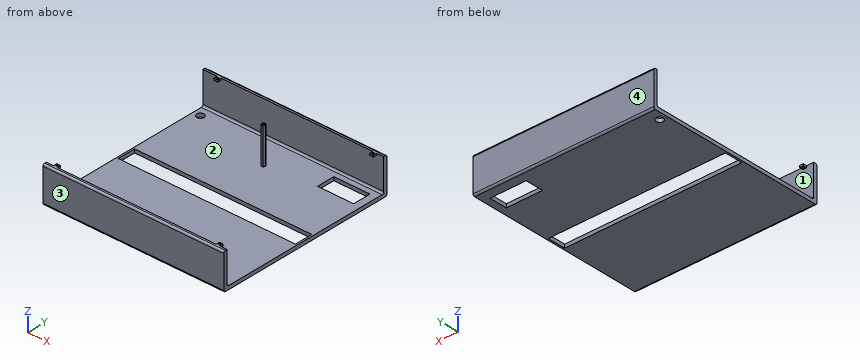
```python
from build123d import *

# Parameters (mm, degrees)
CROQUIS1_W              = 50
CROQUIS1_H              = 50
SALIENTE_EXTRUIR1_DEPTH = 10
CROQUIS2_W              = 49
CROQUIS2_H              = 5
CORTAR_EXTRUIR2_DEPTH   = 6
CROQUIS3_W              = 10
CROQUIS3_H              = 5
CORTAR_EXTRUIR3_DEPTH   = 6
CROQUIS4_R              = 1
CORTAR_EXTRUIR4_DEPTH   = 6
CROQUIS5_W              = 9
CROQUIS5_H              = 48
CORTAR_EXTRUIR5_DEPTH   = 50
CROQUIS6_W              = 1
CROQUIS6_H              = 0.5
SALIENTE_EXTRUIR2_DEPTH = 1
CROQUIS7_W              = 1
CROQUIS7_H              = 0.5
SALIENTE_EXTRUIR3_DEPTH = 1
CROQUIS9_W              = 1
CROQUIS9_H              = 0.5
SALIENTE_EXTRUIR4_DEPTH = 1
CROQUIS10_W             = 1
CROQUIS10_H             = 0.5
SALIENTE_EXTRUIR5_DEPTH = 1
SALIENTE_EXTRUIR6_DEPTH = 10
CROQUIS12_R             = 0.35
CORTAR_EXTRUIR6_DEPTH   = 9
CROQUIS13_R             = 0.25
CORTAR_EXTRUIR7_DEPTH   = 2
CROQUIS14_R             = 0.25
CORTAR_EXTRUIR8_DEPTH   = 2
CROQUIS15_R             = 0.25
CORTAR_EXTRUIR9_DEPTH   = 2
CROQUIS16_R             = 0.25
CORTAR_EXTRUIR10_DEPTH  = 2
REDONDEO5_R             = 0.5
REDONDEO6_R             = 0.5
REDONDEO7_R             = 0.5
REDONDEO8_R             = 0.5
REDONDEO9_R             = 0.5
REDONDEO10_R            = 0.5


with BuildPart() as part:
    # Croquis1 → Saliente-Extruir1 (new body)
    with BuildSketch(Plane.XY):
        Rectangle(CROQUIS1_W, CROQUIS1_H)
    extrude(amount=SALIENTE_EXTRUIR1_DEPTH)

    # Croquis2 → Cortar-Extruir2 (cut)
    with BuildSketch(Plane(origin=(0, 0, 0), x_dir=(-1, 0, 0), z_dir=(0, 0, -1))):
        Rectangle(CROQUIS2_W, CROQUIS2_H)
    extrude(amount=-CORTAR_EXTRUIR2_DEPTH, mode=Mode.SUBTRACT)

    # Croquis3 → Cortar-Extruir3 (cut)
    with BuildSketch(Plane(origin=(0, 0, 0), x_dir=(-1, 0, 0), z_dir=(0, 0, -1))):
        with Locations((-18, 19.5)):
            Rectangle(CROQUIS3_W, CROQUIS3_H)
    extrude(amount=-CORTAR_EXTRUIR3_DEPTH, mode=Mode.SUBTRACT)

    # Croquis4 → Cortar-Extruir4 (cut)
    with BuildSketch(Plane(origin=(0, 0, 0), x_dir=(-1, 0, 0), z_dir=(0, 0, -1))):
        with Locations((23, 21)):
            Circle(CROQUIS4_R)
    extrude(amount=-CORTAR_EXTRUIR4_DEPTH, mode=Mode.SUBTRACT)

    # Croquis5 → Cortar-Extruir5 (cut)
    with BuildSketch(Plane(origin=(25, 0, 0), x_dir=(0, 0, -1), z_dir=(1, 0, 0))):
        with Locations((-5.5, 0)):
            Rectangle(CROQUIS5_W, CROQUIS5_H)
    extrude(amount=-CORTAR_EXTRUIR5_DEPTH, mode=Mode.SUBTRACT)

    # Croquis6 → Saliente-Extruir2 (add)
    with BuildSketch(Plane.XZ.offset(-24)):
        with Locations((-20.5, 9.75)):
            Rectangle(CROQUIS6_W, CROQUIS6_H)
    extrude(amount=SALIENTE_EXTRUIR2_DEPTH)

    # Croquis7 → Saliente-Extruir3 (add)
    with BuildSketch(Plane.XZ.offset(-24)):
        with Locations((22.5, 9.75)):
            Rectangle(CROQUIS7_W, CROQUIS7_H)
    extrude(amount=SALIENTE_EXTRUIR3_DEPTH)

    # Croquis9 → Saliente-Extruir4 (add)
    with BuildSketch(Plane(origin=(0, -24, 0), x_dir=(1, 0, 0), z_dir=(0, 1, 0))):
        with Locations((-22.5, -9.75)):
            Rectangle(CROQUIS9_W, CROQUIS9_H)
    extrude(amount=SALIENTE_EXTRUIR4_DEPTH)

    # Croquis10 → Saliente-Extruir5 (add)
    with BuildSketch(Plane(origin=(0, -24, 0), x_dir=(1, 0, 0), z_dir=(0, 1, 0))):
        with Locations((22.5, -9.75)):
            Rectangle(CROQUIS10_W, CROQUIS10_H)
    extrude(amount=SALIENTE_EXTRUIR5_DEPTH)

    # Croquis11 → Saliente-Extruir6 (add)
    with BuildSketch(Plane.XY.offset(1)):
        Polygon((0, 15.5), (-0.288675135, 16), (-0.866025404, 16), (-1.154700538, 15.5), (-0.866025404, 15), (-0.288675135, 15), align=None)
    extrude(amount=SALIENTE_EXTRUIR6_DEPTH)

    # Croquis12 → Cortar-Extruir6 (cut)
    with BuildSketch(Plane.XY.offset(11)):
        with Locations((-0.6, 15.5)):
            Circle(CROQUIS12_R)
    extrude(amount=-CORTAR_EXTRUIR6_DEPTH, mode=Mode.SUBTRACT)

    # Croquis13 → Cortar-Extruir7 (cut)
    with BuildSketch(Plane.XY.offset(10)):
        with Locations((-20.5, 23.5)):
            Circle(CROQUIS13_R)
    extrude(amount=-CORTAR_EXTRUIR7_DEPTH, mode=Mode.SUBTRACT)

    # Croquis14 → Cortar-Extruir8 (cut)
    with BuildSketch(Plane.XY.offset(10)):
        with Locations((22.5, 23.5)):
            Circle(CROQUIS14_R)
    extrude(amount=-CORTAR_EXTRUIR8_DEPTH, mode=Mode.SUBTRACT)

    # Croquis15 → Cortar-Extruir9 (cut)
    with BuildSketch(Plane.XY.offset(10)):
        with Locations((-22.5, -23.5)):
            Circle(CROQUIS15_R)
    extrude(amount=-CORTAR_EXTRUIR9_DEPTH, mode=Mode.SUBTRACT)

    # Croquis16 → Cortar-Extruir10 (cut)
    with BuildSketch(Plane.XY.offset(10)):
        with Locations((22.5, -23.5)):
            Circle(CROQUIS16_R)
    extrude(amount=-CORTAR_EXTRUIR10_DEPTH, mode=Mode.SUBTRACT)

    # Redondeo5
    redondeo5_edges = [part.edges().sort_by_distance(p)[0] for p in [
        (0, 25, 0),
    ]]
    fillet(redondeo5_edges, radius=REDONDEO5_R)

    # Redondeo6
    redondeo6_edges = [part.edges().sort_by_distance(p)[0] for p in [
        (0, -25, 0),
    ]]
    fillet(redondeo6_edges, radius=REDONDEO6_R)

    # Redondeo7
    redondeo7_edges = [part.edges().sort_by_distance(p)[0] for p in [
        (0, 24, 1),
    ]]
    fillet(redondeo7_edges, radius=REDONDEO7_R)

    # Redondeo8
    redondeo8_edges = [part.edges().sort_by_distance(p)[0] for p in [
        (0, -24, 1),
    ]]
    fillet(redondeo8_edges, radius=REDONDEO8_R)

    # Redondeo9
    redondeo9_edges = [part.edges().sort_by_distance(p)[0] for p in [
        (0, 25, 10),
    ]]
    fillet(redondeo9_edges, radius=REDONDEO9_R)

    # Redondeo10
    redondeo10_edges = [part.edges().sort_by_distance(p)[0] for p in [
        (0, -25, 10),
    ]]
    fillet(redondeo10_edges, radius=REDONDEO10_R)


solid = part.part
```
The listing builds one solid part. Answer for the finished solid, in the listing's coordinates (mm). Face numbers are marked on the shaded views. Give positions to 0.01 mm unless a question says otherwise; leave off trailing zeros. Order: outer loops, then holes, each group sorted by start corner. A loop starts at its lowest first (then second) coordinate and runs counter-clockwise, first axis right, second up.
Item 1: The part is cut by section B-B, the plane z = 4.75. Give the vertices of the cut face in (x, y).
From the geometry:
outline: (-25, -25) - (25, -25) - (25, -24) - (-25, -24) - close; (-25, 24) - (25, 24) - (25, 25) - (-25, 25) - close; (-1.15, 15.5) - (-0.87, 15) - (-0.29, 15) - (0, 15.5) - (-0.29, 16) - (-0.87, 16) - close; hole circle Ø0.7 at (-0.6, 15.5)
Item 2: For a pull along Y with two mould halves and no side action, classify the marked faces 1, 2, 3 and 4 as pulls with the +Y half, pulls with the -Y half, needs draft (parallel to the pull), parting line crosses it, or undercut.
From the geometry:
face 1: undercut
face 2: undercut
face 3: pulls with the -Y half
face 4: pulls with the +Y half
Item 3: The part is cut by section D-D, the plane y = -20.5. Give the vertices of the cut face in (x, z).
From the geometry:
outline: (-25, 0) - (25, 0) - (25, 1) - (-25, 1) - close
Item 4: The part is cut by section A-A, the plane y = 0. Give the vertices of the cut face in (x, z), and give its area (3 significant figures).
From the geometry:
outline: (-25, 0) - (-24.5, 0) - (-24.5, 1) - (-25, 1) - close; (24.5, 0) - (25, 0) - (25, 1) - (24.5, 1) - close
area: 1.00 mm2
Item 5: Given pin 1 Ø1.5 at (y, z) = (16, 9.5) entering from +X, flat-ended and moving along its own axis, determine where the tip first touches the part or whether it passes through.
From the geometry:
pin 1: stops at x = 0
Item 6: Find the intervals of material crossed by probe 1 along Y at (x, z) = (-0.6, 9); probe 2 along X at (y, z) = (23.5, 9.7); probe 3 along Y at (x, z) = (-0.5, 1.75), in increasing order.
From the geometry:
probe 1: y = -25 to -24, 15 to 15.15, 15.85 to 16, 24 to 25
probe 2: x = -21 to -20.75, -20.25 to -20, 22 to 22.25, 22.75 to 23
probe 3: y = -25 to -24, 15 to 16, 24 to 25
Item 7: The part is cut by section C-C, the plane x = -11.5. Give the vertices of the cut face in (y, z), and give its area (3 significant figures).
From the geometry:
outline: (-25, 0.5) arc R0.5 ccw to (-24.5, 0) - (-2.5, 0) - (-2.5, 1) - (-23.5, 1) arc R0.5 cw to (-24, 1.5) - (-24, 10) - (-24.5, 10) arc R0.5 ccw to (-25, 9.5) - close; (2.5, 0) - (24.5, 0) arc R0.5 ccw to (25, 0.5) - (25, 9.5) arc R0.5 ccw to (24.5, 10) - (24, 10) - (24, 1.5) arc R0.5 cw to (23.5, 1) - (2.5, 1) - close
area: 62.9 mm2
